from build123d import *
from build123d.topology import SkipClean

# Parameters (mm, degrees)
BOSS_EXTRUDE1_DEPTH = 34
SKETCH2_R           = 11
BOSS_EXTRUDE2_DEPTH = 2
SKETCH3_R           = 2.5
BOSS_EXTRUDE3_DEPTH = 5.5
BOSS_EXTRUDE4_DEPTH = 16.5


with BuildPart() as part:
    # Sketch1 → Boss-Extrude1 (new body)
    with BuildSketch(Plane(origin=(0, 0, 0), x_dir=(1, 0, 0), z_dir=(0, 1, 0))):
        with BuildLine():
            Line((-15.946583823, -20.203793234), (-17.371924882, -21.629134293))
            Line((-17.371924882, -21.629134293), (-15.371924882, -23.629134293))
            Line((-15.371924882, -23.629134293), (11.828075118, -23.629134293))
            Line((11.828075118, -23.629134293), (13.828075118, -21.629134293))
            Line((13.828075118, -21.629134293), (12.402734059, -20.203793234))
            ThreePointArc((12.402734059, -20.203793234), (9.998571003, -20.203793234), (9.998571003, -17.799630178))
            Line((9.998571003, -17.799630178), (-1.771924882, -6.029134293))
            Line((-1.771924882, -6.029134293), (-13.542420767, -17.799630178))
            ThreePointArc((-13.542420767, -17.799630178), (-13.17390709, -18.351149871), (-13.044502295, -19.001711706))
            ThreePointArc((-13.044502295, -19.001711706), (-14.09394046, -20.572306912), (-15.946583823, -20.203793234))
        make_face()
        with BuildLine():
            Line((-15.946525855, 8.145466679), (-17.371924882, 9.570865707))
            Line((-17.371924882, 9.570865707), (-19.371924882, 7.570865707))
            Line((-19.371924882, 7.570865707), (-19.371924882, -19.629134293))
            Line((-19.371924882, -19.629134293), (-17.371924882, -21.629134293))
            Line((-17.371924882, -21.629134293), (-15.946583823, -20.203793234))
            ThreePointArc((-15.946583823, -20.203793234), (-15.946583823, -17.799630178), (-13.542420767, -17.799630178))
            Line((-13.542420767, -17.799630178), (-1.771924882, -6.029134293))
            Line((-1.771924882, -6.029134293), (-13.542362799, 5.741303623))
            ThreePointArc((-13.542362799, 5.741303623), (-15.946525855, 5.741303623), (-15.946525855, 8.145466679))
        make_face()
        with BuildLine():
            Line((15.828075118, 7.570865707), (13.828075118, 9.570865707))
            Line((13.828075118, 9.570865707), (12.457579233, 8.200369822))
            ThreePointArc((12.457579233, 8.200369822), (12.82609291, 7.648850129), (12.955497705, 6.998288294))
            ThreePointArc((12.955497705, 6.998288294), (11.90605954, 5.427693088), (10.053416177, 5.796206766))
            Line((10.053416177, 5.796206766), (-1.771924882, -6.029134293))
            Line((-1.771924882, -6.029134293), (9.998571003, -17.799630178))
            ThreePointArc((9.998571003, -17.799630178), (11.851214366, -17.431116501), (12.900652531, -19.001711706))
            ThreePointArc((12.900652531, -19.001711706), (12.771247736, -19.652273541), (12.402734059, -20.203793234))
            Line((12.402734059, -20.203793234), (13.828075118, -21.629134293))
            Line((13.828075118, -21.629134293), (15.828075118, -19.629134293))
            Line((15.828075118, -19.629134293), (15.828075118, 7.570865707))
        make_face()
        with BuildLine():
            Line((11.828075118, 11.570865707), (-15.371924882, 11.570865707))
            Line((-15.371924882, 11.570865707), (-17.371924882, 9.570865707))
            Line((-17.371924882, 9.570865707), (-15.946525855, 8.145466679))
            ThreePointArc((-15.946525855, 8.145466679), (-14.093882492, 8.513980357), (-13.044444327, 6.943385151))
            ThreePointArc((-13.044444327, 6.943385151), (-13.173849122, 6.292823316), (-13.542362799, 5.741303623))
            Line((-13.542362799, 5.741303623), (-1.771924882, -6.029134293))
            Line((-1.771924882, -6.029134293), (10.053416177, 5.796206766))
            ThreePointArc((10.053416177, 5.796206766), (10.053416177, 8.200369822), (12.457579233, 8.200369822))
            Line((12.457579233, 8.200369822), (13.828075118, 9.570865707))
            Line((13.828075118, 9.570865707), (11.828075118, 11.570865707))
        make_face()
    extrude(amount=BOSS_EXTRUDE1_DEPTH)

    # Sketch2 → Boss-Extrude2 (add)
    with BuildSketch(Plane(origin=(0, 34, 0), x_dir=(1, 0, 0), z_dir=(0, 1, 0))):
        with Locations(Location((-1.771924882, -6.029134293, 0), (0, 0, 270))):
            Circle(SKETCH2_R)
    extrude(amount=BOSS_EXTRUDE2_DEPTH)

    # Sketch3 → Boss-Extrude3 (add)
    with BuildSketch(Plane(origin=(0, 36, 0), x_dir=(1, 0, 0), z_dir=(0, 1, 0))):
        with Locations(Location((-1.771924882, -6.029134293, 0), (0, 0, 270))):
            Circle(SKETCH3_R)
    extrude(amount=BOSS_EXTRUDE3_DEPTH)

    # Sketch4 → Boss-Extrude4 (add)
    with SkipClean():  # the faces are left unmerged after this step: merging them gives an invalid solid
        with BuildSketch(Plane(origin=(0, 41.5, 0), x_dir=(1, 0, 0), z_dir=(0, 1, 0))):
            with BuildLine():
                Line((-3.271924882, -4.029134293), (-0.271924882, -4.029134293))
                ThreePointArc((-0.271924882, -4.029134293), (-1.771924882, -8.529134293), (-3.271924882, -4.029134293))
            make_face()
        extrude(amount=BOSS_EXTRUDE4_DEPTH)
    add(part.part.scale(1), mode=Mode.REPLACE)  # the faces are merged on a copy


solid = part.part
Part model, mm, in its own coordinate system. A direction names the side the tool comes from. Coordinates: 2 decimals unless noted, no trailing zeros. Write each loop counter-clockwise with the first axis right and the second up, starting at its lowest first coordinate (ties: lowest second). Pieces come first, ordered by that corner, then holes. Notation, with made-up numbers: M 77.5,64.25 L 93.5,64.25 A30 cw 93.5,88.25 Z; hole C 10.25,29.25 d7. An arc over 180 degrees is marked long. Return JSON: item names as keys, results as strings.
1. Flat gauge pins, fed straight in: pin 1 Ø1.5 at (x, z) = (11, 0) entering from +Y; pin 2 Ø4 at (y, z) = (47.5, 4.5) entering from +X; pin 3 Ø0.9 at (x, y) = (-2.5, 48.5) entering from -Z. Where does each tip first touch, or does it go through?
Determined:
{"pin 1": "y = 34", "pin 2": "x = 0.73", "pin 3": "z = 4.03"}
2. Saw through at D-D, the plane x = 1.5. Write the cut outline in (y, z).
Determined:
{"outline": "M 0,-11.57 L 34,-11.57 L 34,-4.47 L 36,-4.47 L 36,16.53 L 34,16.53 L 34,23.63 L 0,23.63 Z"}
3. Saw through at A-A, the plane y = 33. Write the cut outline in (x, z), then the cut area to 3 significant figures.
Determined:
{"outline": "M -19.37,-7.57 L -15.37,-11.57 L 11.83,-11.57 L 15.83,-7.57 L 15.83,19.63 L 11.83,23.63 L -15.37,23.63 L -19.37,19.63 Z; hole C -14.74,-6.94 d3.4; hole C -14.74,19 d3.4; hole C 11.2,19 d3.4; hole C 11.26,-7 d3.4", "area": "1,170 mm²"}
4. 3-axis set-ups, long thin cutter, end or side, ignore diameter. For faces 1 (the face through (-2, 50, 4.029)), 2 (the face through (15.828, 17, 6)), 3 (the face through (-5.985, 34.986, 16.19)): which of +Z, -Z, +X, -X, +Y, -Y reach the whole face in a straight line?
Determined:
{"face 1": "-Z, +X, -X, +Y", "face 2": "+Z, -Z, +X, +Y, -Y", "face 3": "+Y"}
5. Probe L1, parallel to Z at x = -13.5, y = 4.5; L2, parallel to X at y = 12.5, z = -6.5; L3, parallel to Y at x = -12.5, z = 1.5. List the from-to ranges inside material, lowest first.
Determined:
{"L1": "-11.57 to -8.1, -5.79 to 17.84, 20.16 to 23.63", "L2": "-19.37 to -16.39, -13.1 to 9.63, 12.88 to 15.83", "L3": "0 to 34"}
6. Saw through at B-B, the plane x = -14.5. Write the cut outline in (y, z).
Determined:
{"outline": "M 0,-11.57 L 34,-11.57 L 34,-8.63 L 0,-8.63 Z; M 0,-5.26 L 34,-5.26 L 34,17.32 L 0,17.32 Z; M 0,20.68 L 34,20.68 L 34,23.63 L 0,23.63 Z"}
7. Saw through at C-C, the plane z = 7. Write the cut outline in (x, y).
Determined:
{"outline": "M -19.37,0 L 15.83,0 L 15.83,34 L 9.19,34 L 9.19,36 L 0.53,36 L 0.53,58 L -4.08,58 L -4.08,36 L -12.73,36 L -12.73,34 L -19.37,34 Z"}
